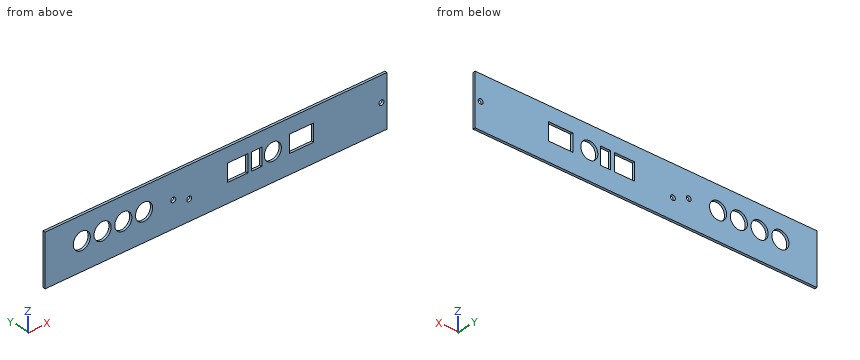
from build123d import *

# Parameters (mm, degrees)
SKETCH_1_W      = 280
SKETCH_1_H      = 41
SKETCH_1_R      = 7
SKETCH_1_R_2    = 2
SKETCH_1_W_2    = 16.5
SKETCH_1_H_2    = 14
SKETCH_1_W_3    = 8.5
SKETCH_1_W_4    = 20
EXTRUDE_1_DEPTH = 2


with BuildPart() as part:
    # 草图1 → 凸台-拉伸1 (new body)
    with BuildSketch(Plane(origin=(0, 0, 0), x_dir=(1, 0, 0), z_dir=(0, 1, 0))):
        with Locations((140, 20.5)):
            Rectangle(SKETCH_1_W, SKETCH_1_H)
        with Locations((30, 18.7)):
            Circle(SKETCH_1_R, mode=Mode.SUBTRACT)
        with Locations((47, 18.7)):
            Circle(SKETCH_1_R, mode=Mode.SUBTRACT)
        with Locations((64, 18.7)):
            Circle(SKETCH_1_R, mode=Mode.SUBTRACT)
        with Locations((81, 18.7)):
            Circle(SKETCH_1_R, mode=Mode.SUBTRACT)
        with Locations((186.5, 18.7)):
            Circle(SKETCH_1_R, mode=Mode.SUBTRACT)
        with Locations((118, 24.7)):
            Circle(SKETCH_1_R_2, mode=Mode.SUBTRACT)
        with Locations((105, 20)):
            Circle(SKETCH_1_R_2, mode=Mode.SUBTRACT)
        with Locations((275.5, 20)):
            Circle(SKETCH_1_R_2, mode=Mode.SUBTRACT)
        with Locations((157.75, 18.7)):
            Rectangle(SKETCH_1_W_2, SKETCH_1_H_2, mode=Mode.SUBTRACT)
        with Locations((173.25, 18.7)):
            Rectangle(SKETCH_1_W_3, SKETCH_1_H_2, mode=Mode.SUBTRACT)
        with Locations((210, 18.7)):
            Rectangle(SKETCH_1_W_4, SKETCH_1_H_2, mode=Mode.SUBTRACT)
    extrude(amount=EXTRUDE_1_DEPTH)


solid = part.part
Can you work these out from the model? Positions are in its coordinate system, mm. Coordinates: 2 decimals unless noted, no trailing zeros. Write each loop counter-clockwise with the first axis right and the second up, starting at its lowest first coordinate (ties: lowest second). Pieces come first, ordered by that corner, then holes. Notation, with made-up numbers: (40, 5) -> (48, 5) arc R11 cw to (48, 19) -> close; hole circle Ø10 at (-34, 77.25). An arc over 180 degrees is marked (long way). Write each question's results on one line, items separated by ' | '. Start each with the question number.
Item 1: If we section it at A-A, the plane y = 0.7: Count the separate pieces of the cut face and the enclosed holes in it, and give its area (3 significant figures).
Item 2: Please list where these lines run through material, in increasing order: probe 1 along Z at (x, y) = (275.5, 1.6); probe 2 along Z at (x, y) = (30, 1.45).
Item 3: I'm going to push a flat-ended pin straight in: P1, Ø12.5, axis at x = 186.5, z = -18.7, coming from the -Y side. Where does the tip first touch, or does it pass through?
Item 4: If we section it at B-B, the plane x = 47: Write out the boundary of the cut face in (y, z), and give its area (3 significant figures).
Answer block:
1) separate pieces: 1 | enclosed holes: 11 | area: 10,000 mm²
2) probe 1: -41 to -22, -18 to 0 | probe 2: -41 to -25.7, -11.7 to 0
3) P1: through
4) outline: (0, -41) -> (2, -41) -> (2, -25.7) -> (0, -25.7) -> close; (0, -11.7) -> (2, -11.7) -> (2, 0) -> (0, 0) -> close | area: 54.0 mm²
